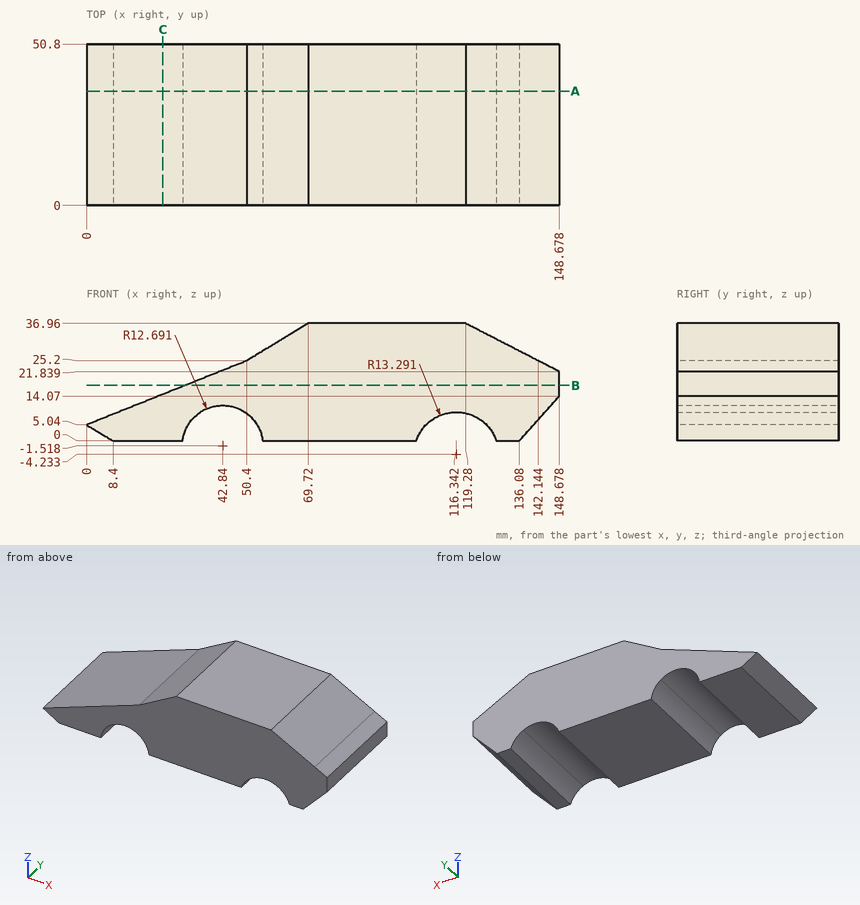
Geometry: see drawing. Coordinates: mm, zero at the bounding-box minimum. Round coordinates to 2 decimals unless told otherwise and drop trailing zeros. Loops run counter-clockwise (first coordinate to the right, second up) from the corner with the lowest first, then second, coordinate; pieces in that order, holes last. Notation, with made-up numbers: (-24.75, 34) - (24.25, 34) arc R24 cw to (24.25, 68) - close; hole circle Ø11 at (-36, 48). An arc over 180 degrees is marked (long way). Write item = value, one per line. Start each with the question number.
(1) Pin query (flat end, axial travel): pin 1 (1.5 mm diameter, centred on y = 44.5, z = 16, fed in from -X) (1 decimal); pin 2 (6 mm diameter, centred on y = 33.5, z = 6.5, fed in from +X) (1 decimal); pin 3 (5 mm diameter, centred on y = 20.5, z = 9.5, fed in from -X); pin 4 (1.5 mm diameter, centred on x = 106.5, z = 14, fed in from -Y). Return the tip coordinate at first contact, or that it passes through.
(2) Section query A-A, the plane y = 36. Output: boundary loops of the cut face in (x, z) (1 decimal).
(3) Section query B-B, the plane z = 17.5. Output: boundary loops of the cut face in (x, y), plus the area to 3 significant figures.
(4) Ray query, line 1 along Z through (x, y) = (116, 33.5); line 2 along X through (y, z) = (3, 15) (1 decimal); line 3 along X through (y, z) = (17, 13) (1 decimal). Return the intervals inside material, ascending. Write a range as from..to.
(5) Section query C-C, the plane x = 24. Output: boundary loops of the cut face in (y, z), plus the area to 3 significant figures.
Conclusion:
q1.pin_1 = 25.5
q1.pin_2 = 144.6
q1.pin_3 = 4.9
q1.pin_4 = 0
q2.outline = (0, 5) - (8.4, 0) - (30.2, 0) arc R12.7 cw to (50.4, 8.7) arc R12.7 cw to (55.4, 0) - (103.7, 0) arc R13.3 cw to (122.4, 7.6) arc R13.3 cw to (128.9, 0) - (136.1, 0) - (148.7, 14.1) - (148.7, 21.8) - (142.1, 25.2) - (119.3, 37) - (69.7, 37) - (50.4, 25.2) - close
q3.outline = (31.15, 0) - (148.68, 0) - (148.68, 50.8) - (31.15, 50.8) - close
q3.area = 5,970 mm2
q4.line_1 = 9.05..36.96
q4.line_2 = 24.9..148.7
q4.line_3 = 19.9..147.7
q5.outline = (0, 0) - (50.8, 0) - (50.8, 14.64) - (0, 14.64) - close
q5.area = 744 mm2
